Autodesk Fusion 360 part; units mm, degrees
sketch "Sketch1" plane through (0, 0, 0) normal (0, 1, 0) x (1, 0, 0)
  line L0 (0, 0) -> (69.24, 0)
  line L1 (69.24, 0) -> (69.24, -69.24)
  line L2 (69.24, -69.24) -> (0, -69.24)
  line L3 (0, -69.24) -> (0, 0)
  dimension "d1" = 69.24
  dimension "d2" = 69.24
extrude "Extrude1" add sketch "Sketch1" along normal blind 5.08
sketch "Sketch2" plane through (0, 0, 0) normal (0, -1, 0) x (1, 0, 0)
  line L0 (69.24, 69.24) -> (0, 69.24)
  line L1 (0, 69.24) -> (0, 0)
  line L2 (0, 0) -> (69.24, 0)
  line L3 (69.24, 0) -> (69.24, 69.24)
  line L4 (-5.38, 74.62) -> (74.62, 74.62)
  line L5 (74.62, 74.62) -> (74.62, -5.38)
  line L6 (74.62, -5.38) -> (-5.38, -5.38)
  line L7 (-5.38, -5.38) -> (-5.38, 74.62)
  point P0 (34.62, 69.24)
  point P1 (34.62, 74.62)
  point P2 (0, 34.62)
  point P3 (-5.38, 34.62)
  dimension "d5" = 80
  dimension "d6" = 80
extrude "Extrude2" add sketch "Sketch2" along normal blind 12.7 contours L0 L1 L2 L3 | L4 L5 L6 L7
fillet "Fillet1" radius 12.7 8 edges at (-5.38, -6.35, 74.62) (74.62, -6.35, 74.62) (74.62, -6.35, -5.38) (-5.38, -6.35, -5.38) (34.62, -12.7, 74.62) (-5.38, -12.7, 34.62) (74.62, -12.7, 34.62) (34.62, -12.7, -5.38)
sketch "Sketch4" plane through (0, -12.7, 0) normal (0, -1, 0) x (1, 0, 0)
  line L0 (7.32, 7.32) -> (61.92, 7.32)
  line L1 (61.92, 7.32) -> (61.92, 61.92)
  line L2 (61.92, 61.92) -> (7.32, 61.92)
  line L3 (7.32, 61.92) -> (7.32, 7.32)
  circle A0 centre (34.62, 34.62) radius 11.938
  dimension "d18" = 23.876
extrude "Extrude4" cut sketch "Sketch4" against normal up to surface (17.78 mm away) contours A0
sketch "Sketch5" plane through (0, 5.08, 0) normal (0, 1, 0) x (-1, 0, 0)
  circle A0 centre (-34.62, 34.62) radius 11.938
  line L0 (0, 69.24) -> (-69.24, 69.24)
  line L1 (-69.24, 69.24) -> (-69.24, 0)
  line L2 (-69.24, 0) -> (0, 0)
  line L3 (0, 0) -> (0, 69.24)
  circle A1 centre (-34.62, 34.62) radius 25
  line L4 (-69.24, 54.62) -> (0, 54.62)
  line L5 (0, 54.62) -> (0, 14.62)
  line L6 (0, 14.62) -> (-69.24, 14.62)
  line L7 (-69.24, 14.62) -> (-69.24, 54.62)
  line L8 (-69.24, 54.62) -> (0, 14.62) construction
  line L9 (0, 54.62) -> (-69.24, 14.62) construction
  point P0 (-34.62, 34.62)
  dimension "d21" = 50
  dimension "d24" = 40
extrude "Extrude5" cut sketch "Sketch5" against normal blind 13.78 contours L3 A1 L4 L5 L6 | L1 A1 L4 L6 L7 | A1 L4 | A1 L4 L6 | A1 L6
ref_plane "WorkPlane2" through (34.62, 2.54, -7.62) normal (0, 0, -1) x (-1, 0, 0)
sketch "Sketch7" plane through (0, 0, -7.62) normal (0, 0, -1) x (-1, 0, 0)
  line L0 (-61.92, 0) -> (-7.32, 0)
  circle A0 centre (-34.62, 0) radius 5.08
  dimension "d28" = 10.16
extrude "Extrude6" cut sketch "Sketch7" against normal blind 5.08 contours L0 A0 picked at (-34.2432, -1.6509)
equation "d1 = 8 cm - 0.4 in - 0.6 mm"
equation "d2 = 8 cm - 0.4 in - 0.6 mm"
equation "d22 = -( 0.7 in - 0.4 cm )"
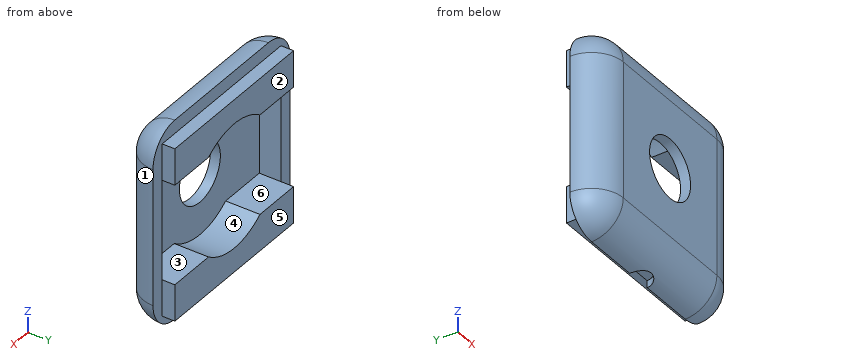
CAD build for the part. Positions are in the model's coordinates, mm. Face numbers are marked on the shaded views. A direction names the side the tool comes from. Round coordinates to 2 decimals unless told otherwise and drop trailing zeros. Write each loop counter-clockwise with the first axis right and the second up, starting at its lowest first coordinate (ties: lowest second). Pieces come first, ordered by that corner, then holes. Notation, with made-up numbers: M -19,29 L 37,29 A20 ccw 37,45 Z; hole C 86.25,35 d1. An arc over 180 degrees is marked long. Use a Markdown table: item, result. Add a question column.
1. Drill centre lines: probe 1 along Y at (x, z) = (9, 29); probe 2 along Z at (x, y) = (38, -8.5); probe 3 along Y at (x, z) = (62.5, 61). Where is each one in solid material? Low to high.
2. Slice it at D-D on y = -10.25. Give the cut face in (x, z).
3. Flat gauge pins, fed straight in: P1, Ø5.5, axis at x = 35, y = -2, coming from the -Z side; P2, Ø3, axis at y = 2.5, z = 50, coming from the +X side; P3, Ø1.5, axis at y = 1.5, z = 4, coming from the +X side; P4, Ø4, axis at x = 9, y = -0.5, coming from the +Z side. Where does each tip first touch, or does it go through?
4. 3-axis set-ups, long thin cutter, end or side, ignore diameter. For the marked faces 5 and 6: which of +Z, -Z, +X, -X, +Y, -Y reach the whole face in a straight line?
5. Slice it at A-A on y = 1.5. Give the cut face in (x, z), then the cut area to 3 significant figures.
6. Pull direction X, two halves, no side cores. Call the marked faces 1, 2, 3 and 4: released by +X, released by -X, zero draft, split by the parting line, or undercut.
Reply:
| question | item | result |
|---|---|---|
| 1 | probe 1 | y = -12.7 to -8.7 |
| 1 | probe 2 | z = -2.12 to 9.85, 59.39 to 71.36 |
| 1 | probe 3 | y = -12.69 to 5.08 |
| 2 | outline | M -0.18,7.32 A7.5 ccw 7.32,-0.18 L 61.92,-0.18 A7.5 ccw 69.42,7.32 L 69.42,61.92 A7.5 ccw 61.92,69.42 L 7.32,69.42 A7.5 ccw -0.18,61.92 Z; hole C 34.62,34.62 d23.88 |
| 3 | P1 | stops at z = -2.54 |
| 3 | P2 | passes through |
| 3 | P3 | stops at x = 69.24 |
| 3 | P4 | stops at z = 74.62 |
| 4 | face 5 | +Z, -Z, +X, -X, +Y |
| 4 | face 6 | +Y |
| 5 | outline | M 0,0 L 69.24,0 L 69.24,14.62 L 49.62,14.62 A25 cw 19.62,14.62 L 0,14.62 Z; M 0,54.62 L 19.62,54.62 A25 cw 49.62,54.62 L 69.24,54.62 L 69.24,69.24 L 0,69.24 Z |
| 5 | area | 1,820 mm^2 |
| 6 | face 1 | released by +X |
| 6 | face 2 | zero draft |
| 6 | face 3 | undercut |
| 6 | face 4 | undercut |
